Input: dimensioned drawing with shaded views. Units: mm. Origin: part minimum x, y, z. A direction names the side the tool comes from. Give positions to 0.01 mm unless a question says otherwise; leave off trailing zeros. Write each loop counter-clockwise with the first axis right and the second up, starting at its lowest first coordinate (ties: lowest second). Pieces come first, ordered by that corner, then holes. Notation, with made-up numbers: (33, 72.25) - (56, 72.25) arc R6 ccw to (56, 77.25) - close; hole circle Ø11 at (71, 64). An arc over 180 degrees is marked (long way). Answer as a JSON object with one key per item and string values. Group by question number.
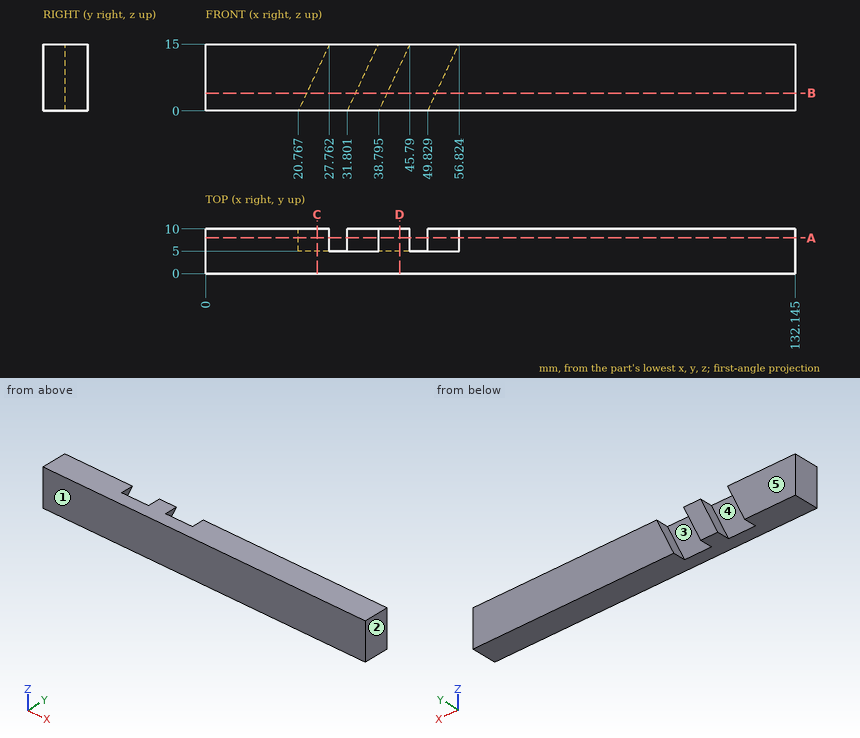
Q1. First-contact query: pin 1 Ø7.5 at (x, z) = (48.5, 9) entering from +Y. Flat tip, straight axial feed; report the tip coordinate or a pass-through.
Q2. Section C-C on x = 25. Return the cut outline in (y, z), then the cut area to 3 significant figures.
Q3. Reachability of the marked faces 4 and 5 from +Z, -Z, +X, -X, +Y, -Y: full face, straight path, thin tool, end or side. Return the list, or none.
Q4. Ray query, probe 1 along X at (y, z) = (5.5, 12.25) (1 decimal); probe 2 along X at (y, z) = (6.75, 3) (1 decimal); probe 3 along Y at (x, z) = (52, 9.5). Return the intervals inside material, ascending. Write a range as [from, to].
Q5. Section A-A on y = 8. Return the cut outline in (x, z) (1 decimal), then the cut area to 3 significant figures.
Q6. Section B-B on z = 4. Return the cut outline in (x, y) (1 decimal), then the cut area to 3 significant figures.
Q7. Draft query along X for the marked faces 1, 2 and 3. Return one class per face: released by +X, released by -X, zero draft, split by the parting line, or undercut.
Q8. Section D-D on x = 43.5. Return the cut outline in (y, z).
Taken from the geometry:
{
 "1": {"pin 1": "stops at y = 5"},
 "2": {"outline": "(0, 0) - (5, 0) - (5, 9.08) - (10, 9.08) - (10, 15) - (0, 15) - close", "area": "105 mm²"},
 "3": {"face 4": "+Y", "face 5": "+Z, -Z, +X, -X, +Y"},
 "4": {"probe 1": "x = [0, 26.5], [37.5, 44.5], [55.5, 132.1]", "probe 2": "x = [0, 22.2], [33.2, 40.2], [51.2, 132.1]", "probe 3": "y = [0, 5]"},
 "5": {"outline": "(0, 0) - (20.8, 0) - (27.8, 15) - (0, 15) - close; (31.8, 0) - (38.8, 0) - (45.8, 15) - (38.8, 15) - close; (49.8, 0) - (132.1, 0) - (132.1, 15) - (56.8, 15) - close", "area": "1,650 mm²"},
 "6": {"outline": "(0, 0) - (132.1, 0) - (132.1, 10) - (51.7, 10) - (51.7, 5) - (40.7, 5) - (40.7, 10) - (33.7, 10) - (33.7, 5) - (22.6, 5) - (22.6, 10) - (0, 10) - close", "area": "1,210 mm²"},
 "7": {"face 1": "zero draft", "face 2": "released by +X", "face 3": "undercut"},
 "8": {"outline": "(0, 0) - (5, 0) - (5, 10.09) - (10, 10.09) - (10, 15) - (0, 15) - close"}
}
